from build123d import *

# Parameters (mm, degrees)
F0_W      = 43.5
F0_H      = 23.5
F1_DEPTH  = 2
F2_W      = 40.5
F2_H      = 20.5
F3_DEPTH  = 5
F4_W      = 35.5
F4_H      = 15.5
F5_DEPTH  = 3
F6_W      = 40.5
F6_H      = 20.5
F7_DEPTH  = 2
F8_R      = 0.5
F9_R      = 1.5
F10_DEPTH = 25


with BuildPart() as f1:
    # F0 (on Top) → F1 (new body)
    with BuildSketch(Plane.XY):
        Rectangle(F0_W, F0_H)
    extrude(amount=F1_DEPTH)

    # F2 (on face) → F3 (join)
    with BuildSketch(Plane.XY.offset(2)):
        Rectangle(F2_W, F2_H)
    extrude(amount=F3_DEPTH)

    # F4 (on face) → F5 (join)
    with BuildSketch(Plane.XY.offset(7)):
        Rectangle(F4_W, F4_H)
    extrude(amount=F5_DEPTH)

    # F6 (on face) → F7 (join)
    with BuildSketch(Plane.XY.offset(10)):
        Rectangle(F6_W, F6_H)
    extrude(amount=F7_DEPTH)

    # F8
    f8_edges = [f1.edges().sort_by_distance(p)[0] for p in [
        (-20.25, 10.25, 4.5),
        (-17.75, 7.75, 8.5),
        (-20.25, 10.25, 11),
        (-20.25, -10.25, 4.5),
        (-17.75, -7.75, 8.5),
        (-20.25, -10.25, 11),
        (20.25, -10.25, 4.5),
        (17.75, -7.75, 8.5),
        (20.25, -10.25, 11),
        (20.25, 10.25, 4.5),
        (17.75, 7.75, 8.5),
        (20.25, 10.25, 11),
        (21.75, -11.75, 1),
        (21.75, 11.75, 1),
        (-21.75, -11.75, 1),
        (-21.75, 11.75, 1),
    ]]
    fillet(f8_edges, radius=F8_R)

    # F9 (on face) → F10 (cut)
    with BuildSketch(Plane.XZ.offset(10.25)):
        with Locations((0, 4.5)):
            Circle(F9_R)
    extrude(amount=-F10_DEPTH, mode=Mode.SUBTRACT)


solid = f1.part
Could you check a few things on this model? Use its own coordinates, in mm. A direction names the side the tool comes from. Give positions to 0.01 mm unless a question says otherwise; leave off trailing zeros. Order: outer loops, then holes, each group sorted by start corner. A loop starts at its lowest first (then second) coordinate and runs counter-clockwise, first axis right, second up. Notation, with made-up numbers: (7.5, -28) - (61.5, -28) arc R9 ccw to (61.5, -14) - close; hole circle Ø1 at (3.5, 58.5). An arc over 180 degrees is marked (long way). One line per item, written item: value. Start each with the question number.
1. Imagine slicing it at D-D on z = 9. List the corners of the cut face in (x, y) for me, plus the area to 3 significant figures.
2. Imagine slicing it at B-B on y = -4.75. List the corners of the cut face in (x, z) for me, plus the area to 3 significant figures.
3. Imagine slicing it at A-A on z = 4.5. List the corners of the cut face in (x, y) for me.
4. Thinking about a two-plate mould opening in Z: for faces 4 (the face through (0, 7.75, 8)), 5 (the face through (-1.7, -10.4, 2)), 6 (the face through (-20.25, 0, 11)), 7 (the face through (17.75, 0, 8)), which applies, +Z half, -Z half, draft (parallel to the pull), parting line (faces both ways), or undercut?
5. Imagine slicing it at C-C on x = 0. List the corners of the cut face in (y, z) for me, plus the area to 4 significant figures.
6. For P1, Ø5.5, axis at y = 0.5, z = 5, coming from the -X side; P2, Ø0.9, axis at y = 0.5, z = 9, coming from the -X side; P3, Ø3, axis at x = -13.5, z = 6, coming from the -Y side, each with a flat end and sliding along its axis, tell me the tip position at first contact or that it passes through.
7. For faces 1 (the face through (0, 8, 7)), 2 (the face through (0, -7.75, 8)), 3 (the face through (-17.75, 0, 8)), which set-ups out of +Z, -Z, +X, -X, +Y, -Y let a thin tool reach every point of the face, with its end or its side?
8. If I drill on probe 1 along Z at (x, y) = (0, 1.75); probe 2 along Z at (x, y) = (-19, -0.5); probe 3 along Y at (x, z) = (-4, 9), over which ranges is the centre line in solid material (lowest first)?
Values:
1. outline: (-17.75, -7.25) arc R0.5 ccw to (-17.25, -7.75) - (17.25, -7.75) arc R0.5 ccw to (17.75, -7.25) - (17.75, 7.25) arc R0.5 ccw to (17.25, 7.75) - (-17.25, 7.75) arc R0.5 ccw to (-17.75, 7.25) - close
1. area: 550 mm²
2. outline: (-21.75, 0) - (21.75, 0) - (21.75, 2) - (20.25, 2) - (20.25, 7) - (17.75, 7) - (17.75, 10) - (20.25, 10) - (20.25, 12) - (-20.25, 12) - (-20.25, 10) - (-17.75, 10) - (-17.75, 7) - (-20.25, 7) - (-20.25, 2) - (-21.75, 2) - close; hole circle Ø3 at (0, 4.5)
2. area: 470 mm²
3. outline: (-20.25, -9.75) arc R0.5 ccw to (-19.75, -10.25) - (-1.5, -10.25) - (-1.5, 10.25) - (-19.75, 10.25) arc R0.5 ccw to (-20.25, 9.75) - close; (1.5, -10.25) - (19.75, -10.25) arc R0.5 ccw to (20.25, -9.75) - (20.25, 9.75) arc R0.5 ccw to (19.75, 10.25) - (1.5, 10.25) - close
4. face 4: undercut
4. face 5: +Z half
4. face 6: draft
4. face 7: undercut
5. outline: (-11.75, 0) - (11.75, 0) - (11.75, 2) - (10.25, 2) - (10.25, 3) - (-10.25, 3) - (-10.25, 2) - (-11.75, 2) - close; (-10.25, 6) - (10.25, 6) - (10.25, 7) - (7.75, 7) - (7.75, 10) - (10.25, 10) - (10.25, 12) - (-10.25, 12) - (-10.25, 10) - (-7.75, 10) - (-7.75, 7) - (-10.25, 7) - close
5. area: 175.5 mm²
6. P1: x = -20.25
6. P2: x = -17.75
6. P3: y = -10.25
7. face 1: none
7. face 2: +X, -X, -Y
7. face 3: -X, +Y, -Y
8. probe 1: 0 to 3, 6 to 12
8. probe 2: 0 to 7, 10 to 12
8. probe 3: -7.75 to 7.75
